```python
from build123d import *

# Parameters (mm, degrees)
F1_DEPTH       = 2
F3_R           = 1.5
F5_DEPTH       = 15
F6_R           = 1.25
F7_DEPTH       = 66
F9_D           = 4.4
F9_DEPTH       = 14.1
F9_CSINK_D     = 8.96
F9_CSINK_ANGLE = 90
F9_TIP         = 1.3218933619


# Not quite as in the source:
# - an extrude ends at something that could not be found from the text; its depth is read off the source's solid


with BuildPart() as f1:
    # F0 (on Top) → F1 (new body)
    with BuildSketch(Plane.XY):
        with BuildLine():
            ThreePointArc((20, 5), (18.5355339059, 8.5355339059), (15, 10))
            Line((15, 10), (-15, 10))
            ThreePointArc((-15, 10), (-18.5355339059, 8.5355339059), (-20, 5))
            Line((-20, 5), (-20, -10))
            Line((-20, -10), (20, -10))
            Line((20, -10), (20, 5))
        make_face()
    extrude(amount=F1_DEPTH)

    # F3 (on offset) → F5 (join, through all)
    with BuildSketch(Plane.YZ.offset(7.5)):
        with Locations((-10, 3.25)):
            Circle(F3_R)
    extrude(amount=-F5_DEPTH)

    # F6 (on face) → F7 (cut, through all)
    with BuildSketch(Plane.YZ.offset(20)):
        with Locations((-10, 3.25)):
            Circle(F6_R)
    extrude(amount=-F7_DEPTH, mode=Mode.SUBTRACT)

    # F9
    with Locations(Plane.XY.offset(2)):
        with Locations((-12.5, 0), (12.5, 0)):
            CounterSinkHole(F9_D / 2, F9_CSINK_D / 2, depth=F9_DEPTH, counter_sink_angle=F9_CSINK_ANGLE)
            with Locations((0, 0, -(F9_DEPTH + F9_TIP / 2))):  # 118° drill point
                Cone(0, F9_D / 2, F9_TIP, mode=Mode.SUBTRACT)


solid = f1.part
```
For this review, take the finished solid that the model builds, in its own axes (mm). Round coordinates to 2 decimals unless told otherwise and drop trailing zeros. Order: outer loops, then holes, each group sorted by start corner. A loop starts at its lowest first (then second) coordinate and runs counter-clockwise, first axis right, second up. Notation, with made-up numbers: (83, -33) -> (126, -33) arc R31 cw to (126, 3) -> close; hole circle Ø7 at (25, 50.5). An arc over 180 degrees is marked (long way). Use a Markdown table: item, result.
Item 1: Take a section at C-C (z = 0.75). State the section outline as (x, y) points, plus the area to 3 significant figures.
Resolved:
| item | result |
|---|---|
| outline | (-20, -10) -> (20, -10) -> (20, 5) arc R5 ccw to (15, 10) -> (-15, 10) arc R5 ccw to (-20, 5) -> close; hole circle Ø6.46 at (-12.5, 0); hole circle Ø6.46 at (12.5, 0) |
| area | 724 mm² |
Item 2: Take a section at A-A (y = 0). State the section outline as (x, z) points.
Resolved:
| item | result |
|---|---|
| outline | (-20, 0) -> (-14.98, 0) -> (-16.98, 2) -> (-20, 2) -> close; (-10.02, 0) -> (10.02, 0) -> (8.02, 2) -> (-8.02, 2) -> close; (14.98, 0) -> (20, 0) -> (20, 2) -> (16.98, 2) -> close |
Item 3: Take a section at D-D (z = 3.25). State the section outline as (x, y) points, plus the area to 3 significant figures.
Resolved:
| item | result |
|---|---|
| outline | (-7.5, -11.5) -> (7.5, -11.5) -> (7.5, -11.25) -> (-7.5, -11.25) -> close; (-7.5, -8.75) -> (7.5, -8.75) -> (7.5, -8.5) -> (-7.5, -8.5) -> close |
| area | 7.50 mm² |
Item 4: For line 1 along Y through (x, z) = (2.75, 3.25); line 2 along X through (y, z) = (-1, 0.85); line 3 along Z through (x, y) = (-1.5, -5), list the stretches that pass through material, from the lowest coordinate up. Write a range as [from, to].
Resolved:
| item | result |
|---|---|
| line 1 | y = [-11.5, -11.25], [-8.75, -8.5] |
| line 2 | x = [-20, -15.68], [-9.32, 9.32], [15.68, 20] |
| line 3 | z = [0, 2] |
Item 5: For pin 1 (1.6 mm diameter, centred on x = 3.5, z = 1.5, fed in from -Y); pin 2 (6 mm diameter, centred on x = 8, y = 0, fed in from +Z); pin 3 (2 mm diameter, centred on x = -13, z = 1, fed in from -Y), all flat-tipped, find the tip position at first contact; note any pin that passes through.
Resolved:
| item | result |
|---|---|
| pin 1 | stops at y = -11.16 |
| pin 2 | stops at z = 2 |
| pin 3 | stops at y = -10 |
Item 6: Draft analysis for pull direction Z (two halves, no side actions). For faces 1 (the cylindrical face through (0.11, -11.25, 3.3)), 2 (the flat face through (-20, -2, 1)), 3 (the flat face through (0, 0, 0)), state which applies: +Z half, -Z half, draft (parallel to the pull), parting line (faces both ways), or undercut.
Resolved:
| item | result |
|---|---|
| face 1 | undercut |
| face 2 | draft |
| face 3 | -Z half |
Item 7: Take a section at B-B (x = -12.5). State the section outline as (y, z) points.
Resolved:
| item | result |
|---|---|
| outline | (-10, 0) -> (-2.48, 0) -> (-4.48, 2) -> (-10, 2) -> close; (2.48, 0) -> (10, 0) -> (10, 2) -> (4.48, 2) -> close |
